from build123d import *

# Parameters (mm, degrees)
EXTRUDE_1_DEPTH     = 16
F_1_0MM_1_D         = 2.6
F_1_0MM_2_D         = 2.6
SKETCH_8_W          = 86.7
SKETCH_8_H          = 16
EXTRUDE_2_DEPTH     = 21.2
SKETCH_9_W          = 86.7
SKETCH_9_H          = 10.4
EXTRUDE_3_DEPTH     = 9.7
SKETCH_15_W         = 20.6
SKETCH_15_H         = 2
EXTRUDE_8_DEPTH     = 13.5
SKETCH_16_W         = 20.6
SKETCH_16_H         = 2
EXTRUDE_9_DEPTH     = 10.5
SKETCH_19_W         = 51.4
SKETCH_19_H         = 10.4
EXTRUDE_10_DEPTH    = 20
SKETCH_25_W         = 20
SKETCH_25_H         = 10.4
EXTRUDE_11_DEPTH    = 45
EXTRUDE_12_DEPTH    = 32
CUT_EXTRUDE_1_DEPTH = 5
SKETCH_29_W         = 51.4
SKETCH_29_H         = 10.402970243
EXTRUDE_13_DEPTH    = 40
SKETCH_32_W         = 40
SKETCH_32_H         = 10.402970243
EXTRUDE_14_DEPTH    = 10
SKETCH_33_W         = 40
SKETCH_33_H         = 10.402970243
EXTRUDE_15_DEPTH    = 10
SKETCH_34_R         = 3
EXTRUDE_16_DEPTH    = 12
F_1_0MM_3_D         = 2.6
F_1_0MM_4_D         = 2.6


with BuildPart() as part:
    # 草图1 → 凸台-拉伸1 (new body)
    with BuildSketch(Plane.XY):
        Polygon((-21.523113208, 25.59839861), (-42.123113208, 25.59839861), (-42.123113208, 5.59839861), (44.576886792, 5.59839861), (44.576886792, 25.59839861), (23.976886792, 25.59839861), (23.976886792, 13.12839861), (-21.523113208, 13.12839861), align=None)
    extrude_1 = extrude(amount=EXTRUDE_1_DEPTH)

    # Ø1.0mm 暗销孔1 (through all)
    with Locations(Plane(origin=(0, 25.59839861, 0), x_dir=(1, 0, 0), z_dir=(0, 1, 0))):
        with Locations((36.576886792, -8)):
            f_1_0mm_1 = Hole(F_1_0MM_1_D / 2)

    # Ø1.0mm 暗销孔2 (through all)
    with Locations(Plane(origin=(0, 25.59839861, 0), x_dir=(1, 0, 0), z_dir=(0, 1, 0))):
        with Locations((-34.123113208, -8)):
            f_1_0mm_2 = Hole(F_1_0MM_2_D / 2)

    # 草图8 → 凸台-拉伸2 (add)
    with BuildSketch(Plane.XZ.offset(-5.59839861)):
        with Locations((1.226886792, 8)):
            Rectangle(SKETCH_8_W, SKETCH_8_H)
    extrude_2 = extrude(amount=EXTRUDE_2_DEPTH)

    # 草图9 → 凸台-拉伸3 (add)
    with BuildSketch(Plane(origin=(0, 0, 0), x_dir=(-1, 0, 0), z_dir=(0, 0, -1))):
        with Locations((-1.226886792, -10.40160139)):
            Rectangle(SKETCH_9_W, SKETCH_9_H)
    extrude_3 = extrude(amount=EXTRUDE_3_DEPTH)

    # 草图15 → 凸台-拉伸8 (add)
    with BuildSketch(Plane(origin=(0, -5.20160139, 0), x_dir=(1, 0, 0), z_dir=(0, 1, 0))):
        with Locations((-31.823113208, 8.7)):
            Rectangle(SKETCH_15_W, SKETCH_15_H)
    extrude_8 = extrude(amount=EXTRUDE_8_DEPTH)

    # 草图16 → 凸台-拉伸9 (add)
    with BuildSketch(Plane(origin=(0, 0, -9.7), x_dir=(-1, 0, 0), z_dir=(0, 0, -1))):
        with Locations((31.823113208, 7.29839861)):
            Rectangle(SKETCH_16_W, SKETCH_16_H)
    extrude_9 = extrude(amount=-EXTRUDE_9_DEPTH)

    # 镜向20: 凸台-拉伸1, Ø1.0mm 暗销孔1, Ø1.0mm 暗销孔2, 凸台-拉伸2, 凸台-拉伸3, 凸台-拉伸8, 凸台-拉伸9 across plane
    add(extrude_1.mirror(Plane.XY.offset(-9.7)))
    add(f_1_0mm_1.mirror(Plane.XY.offset(-9.7)), mode=Mode.SUBTRACT)
    add(f_1_0mm_2.mirror(Plane.XY.offset(-9.7)), mode=Mode.SUBTRACT)
    add(extrude_2.mirror(Plane.XY.offset(-9.7)))
    add(extrude_3.mirror(Plane.XY.offset(-9.7)))
    add(extrude_8.mirror(Plane.XY.offset(-9.7)))
    add(extrude_9.mirror(Plane.XY.offset(-9.7)))

    # 草图19 → 凸台-拉伸10 (add)
    with BuildSketch(Plane(origin=(44.576886792, 0, 0), x_dir=(0, 0, -1), z_dir=(1, 0, 0))):
        with Locations((9.7, -10.40160139)):
            Rectangle(SKETCH_19_W, SKETCH_19_H)
    extrude(amount=EXTRUDE_10_DEPTH)

    # 草图25 → 凸台-拉伸11 (add)
    with BuildSketch(Plane(origin=(0, 0, -35.4), x_dir=(-1, 0, 0), z_dir=(0, 0, -1))):
        with Locations((-54.576886792, -10.40160139)):
            Rectangle(SKETCH_25_W, SKETCH_25_H)
    extrude(amount=EXTRUDE_11_DEPTH)

    # 草图26 → 凸台-拉伸12 (add)
    with BuildSketch(Plane(origin=(0, -5.20160139, 0), x_dir=(1, 0, 0), z_dir=(0, 1, 0))):
        Polygon((53.176886792, -9), (64.576886792, -9), (64.576886792, -5), (64.576886792, 80.4), (60.576886792, 80.4), (60.576886792, -5), (53.176886792, -5), align=None)
        Polygon((53.176886792, 28), (54.576886792, 28), (54.576886792, 68), (53.176886792, 68), (51.776886792, 68), (51.776886792, 28), align=None)
    extrude(amount=EXTRUDE_12_DEPTH)

    # 草图28 → 切除-拉伸1 (cut)
    with BuildSketch(Plane(origin=(0, -5.20160139, 0), x_dir=(1, 0, 0), z_dir=(0, 1, 0))):
        Polygon((60.576886792, 80.4), (54.576886792, 80.4), (54.576886792, 28), (52.576886792, 28), (52.576886792, -5), (54.576886792, -5), (60.576886792, -5), (60.576886792, 28), align=None)
    extrude(amount=-CUT_EXTRUDE_1_DEPTH, mode=Mode.SUBTRACT)

    # 草图29 → 凸台-拉伸13 (add)
    with BuildSketch(Plane.ZY.offset(42.123113208)):
        with Locations((-9.7, -10.400116268)):
            Rectangle(SKETCH_29_W, SKETCH_29_H)
    extrude(amount=EXTRUDE_13_DEPTH)

    # 草图32 → 凸台-拉伸14 (add)
    with BuildSketch(Plane(origin=(0, 0, -35.4), x_dir=(-1, 0, 0), z_dir=(0, 0, -1))):
        with Locations((62.123113208, -10.400116268)):
            Rectangle(SKETCH_32_W, SKETCH_32_H)
    extrude(amount=EXTRUDE_14_DEPTH)

    # 草图33 → 凸台-拉伸15 (add)
    with BuildSketch(Plane.XY.offset(16)):
        with Locations((-62.123113208, -10.400116268)):
            Rectangle(SKETCH_33_W, SKETCH_33_H)
    extrude(amount=EXTRUDE_15_DEPTH)

    # 草图34 → 凸台-拉伸16 (add)
    with BuildSketch(Plane(origin=(0, -5.198631147, 0), x_dir=(1, 0, 0), z_dir=(0, 1, 0))):
        with Locations(Location((-52.123113208, 38.7, 0), (0, 0, 90))):
            Circle(SKETCH_34_R)
        with Locations(Location((-75.123113208, 38.7, 0), (0, 0, 90))):
            Circle(SKETCH_34_R)
        with Locations(Location((-52.123113208, -19.3, 0), (0, 0, 90))):
            Circle(SKETCH_34_R)
        with Locations(Location((-75.123113208, -19.3, 0), (0, 0, 90))):
            Circle(SKETCH_34_R)
    extrude(amount=EXTRUDE_16_DEPTH)

    # Ø1.0mm 暗销孔3 (through all)
    with Locations(Plane(origin=(0, 6.801368853, 0), x_dir=(1, 0, 0), z_dir=(0, 1, 0))):
        with Locations((-52.123113208, 38.7)):
            Hole(F_1_0MM_3_D / 2)

    # Ø1.0mm 暗销孔4 (through all)
    with Locations(Plane(origin=(0, 6.801368853, 0), x_dir=(1, 0, 0), z_dir=(0, 1, 0))):
        with Locations((-52.123113208, -19.3), (-75.123113208, 38.7), (-75.123113208, -19.3)):
            Hole(F_1_0MM_4_D / 2)


solid = part.part
Input: part model. Units: mm. Frame: model coordinates. A direction names the side the tool comes from. Give positions to 0.01 mm unless a question says otherwise; leave off trailing zeros. Write each loop counter-clockwise with the first axis right and the second up, starting at its lowest first coordinate (ties: lowest second). Pieces come first, ordered by that corner, then holes.
Q1. Section B-B, the plane y = 11.5. Output: boundary loops of the cut face in (x, z).
Q2. First-contact query: P1, Ø3, axis at x = 20, z = -38.5, coming from the +Y side; P2, Ø6, axis at y = 11.5, z = -38, coming from the -X side; P3, Ø5, axis at x = -74, z = 18, coming from the +Y side; P4, Ø3, axis at x = -72, y = -8, coming from the -Z side. Flat tips, straight axial feed; report the tip coordinate or a pass-through.
Q3. Material intervals for probe 1 along X at (y, z) = (13, 8); probe 2 along X at (y, z) = (-4.75, -38.7); probe 3 along X at (y, z) = (-0.5, 19.3), sorted ascending.
Q4. Section A-A, the plane y = 20.5. State how many separate pieces and enclosed holes the cut face has, plus the area to 3 significant figures.
Q5. Set-up query: faces 1 (the face through (-32, 0, -7.7)), 2 (the face through (-72.46, 0.72, 17.92)), 3 (the face through (-21.523, 19, -27)), 4 (the face through (0, 0, 16)). Return all of +Z, -Z, +X, -X, +Y, -Y with unobstructed straight access to the full face (end or side cutting, diameter ignored); none if empty.
Q6. Pull-direction query (Y, two-part tool) for faces 5 (the face through (-32, 6.298, -15)), 6 (the face through (-82.123, -10, -10)), 7 (the face through (-32, 25.598, -27)); classes: pulls with the +Y half, pulls with the -Y half, needs draft (parallel to the pull), parting line crosses it, or undercut.
Q7. Section D-D, the plane x = -2.5. Output: boundary loops of the cut face in (y, z), plus the area to 3 significant figures.
Filled in:
1. outline: (-42.12, -35.4) - (44.58, -35.4) - (44.58, -19.4) - (-42.12, -19.4) - close; (-42.12, 0) - (44.58, 0) - (44.58, 16) - (-42.12, 16) - close; (51.78, -68) - (54.58, -68) - (54.58, -28) - (51.78, -28) - close; (53.18, 5) - (60.58, 5) - (60.58, -80.4) - (64.58, -80.4) - (64.58, 9) - (53.18, 9) - close; hole circle Ø2.6 at (-34.12, -27.4); hole circle Ø2.6 at (-34.12, 8); hole circle Ø2.6 at (36.58, -27.4); hole circle Ø2.6 at (36.58, 8)
2. P1: passes through
2. P2: stops at x = -42.12
2. P3: stops at y = 6.8
2. P4: stops at z = -45.4
3. probe 1: x = -42.12 to -35.42, -32.82 to 35.28, 37.88 to 44.58, 53.18 to 64.58
3. probe 2: x = -78.12 to -76.42, -73.82 to -72.12, -55.12 to -53.42, -50.82 to -49.12, 51.78 to 54.58, 60.58 to 64.58
3. probe 3: x = -78.12 to -76.42, -73.82 to -72.12, -55.12 to -53.42, -50.82 to -49.12
4. separate pieces: 6
4. enclosed holes: 4
4. area: 1,800 mm2
5. face 1: -X
5. face 2: +Y
5. face 3: +Z, -Z, +Y
5. face 4: +Z, +X, +Y, -Y
6. face 5: undercut
6. face 6: needs draft
6. face 7: pulls with the +Y half
7. outline: (-15.6, -35.4) - (13.13, -35.4) - (13.13, -19.4) - (-5.2, -19.4) - (-5.2, 0) - (13.13, 0) - (13.13, 16) - (-15.6, 16) - close
7. area: 1,120 mm2
